Verification items for the finished model (mm, model axes). Give positions to 0.01 mm unless a question says otherwise; leave off trailing zeros. Write each loop counter-clockwise with the first axis right and the second up, starting at its lowest first coordinate (ties: lowest second). Pieces come first, ordered by that corner, then holes.
from build123d import *

# Parameters (mm, degrees)
F0_W     = 400
F0_H     = 100
F0_R     = 4.25
F1_DEPTH = 10


with BuildPart() as f1:
    # F0 (on Top) → F1 (new body)
    with BuildSketch(Plane.XY):
        with Locations((97, -30)):
            Rectangle(F0_W, F0_H)
        with Locations((0, -60)):
            Circle(F0_R, mode=Mode.SUBTRACT)
        with Locations((54, -60)):
            Circle(F0_R, mode=Mode.SUBTRACT)
        with Locations((140, -60)):
            Circle(F0_R, mode=Mode.SUBTRACT)
        with Locations((194, -60)):
            Circle(F0_R, mode=Mode.SUBTRACT)
        Circle(F0_R, mode=Mode.SUBTRACT)
        with Locations((54, 0)):
            Circle(F0_R, mode=Mode.SUBTRACT)
        with Locations((140, 0)):
            Circle(F0_R, mode=Mode.SUBTRACT)
        with Locations((194, 0)):
            Circle(F0_R, mode=Mode.SUBTRACT)
    extrude(amount=F1_DEPTH)


solid = f1.part
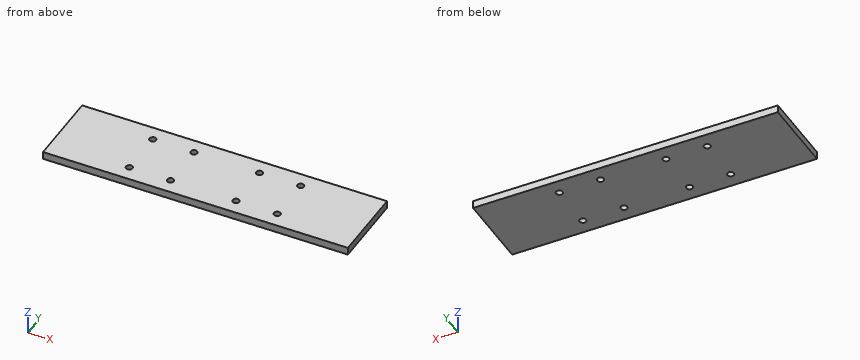
Item 1: Depth check by flat-ended pin: pin 1 (5 mm diameter, centred on x = 194, y = -60, fed in from +Z); pin 2 (12 mm diameter, centred on x = 3.5, y = -60.5, fed in from +Z). Enter the tip coordinate at first touch or a pass-through.
Answer key:
pin 1: passes through
pin 2: stops at z = 10
Item 2: Sectioned sample at A-A on y = -60. Record the cut outline in (x, z).
Answer key:
outline: (-103, 0) - (-4.25, 0) - (-4.25, 10) - (-103, 10) - close; (4.25, 0) - (49.75, 0) - (49.75, 10) - (4.25, 10) - close; (58.25, 0) - (135.75, 0) - (135.75, 10) - (58.25, 10) - close; (144.25, 0) - (189.75, 0) - (189.75, 10) - (144.25, 10) - close; (198.25, 0) - (297, 0) - (297, 10) - (198.25, 10) - close
Item 3: Scan lines: line 1 along Y through (x, z) = (140, 7.75); line 2 along X through (y, z) = (-0.5, 6.75); line 3 along Y through (x, z) = (-2, 3.5). Record each from-to range of solid material in increasing order.
Answer key:
line 1: y = -80 to -64.25, -55.75 to -4.25, 4.25 to 20
line 2: x = -103 to -4.22, 4.22 to 49.78, 58.22 to 135.78, 144.22 to 189.78, 198.22 to 297
line 3: y = -80 to -63.75, -56.25 to -3.75, 3.75 to 20
Item 4: Sectioned sample at B-B on x = 0. Record the cut outline in (y, z).
Answer key:
outline: (-80, 0) - (-64.25, 0) - (-64.25, 10) - (-80, 10) - close; (-55.75, 0) - (-4.25, 0) - (-4.25, 10) - (-55.75, 10) - close; (4.25, 0) - (20, 0) - (20, 10) - (4.25, 10) - close
